```python
from build123d import *

# Parameters (mm, degrees)
BOSS_EXTRUDE4_DEPTH      = 3
SKETCH8_W                = 3
SKETCH8_H                = 8
SKETCH8_H_2              = 14.11
CUT_EXTRUDE5_DEPTH       = 3
SKETCH9_R                = 0.75
SKETCH9_W                = 12
SKETCH9_H                = 23.5
CUT_EXTRUDE6_DEPTH       = 3
FILLET2_R                = 5
SPLIT1_SURFACE_1_1_BACK  = 91.82
SPLIT1_SURFACE_1_1_DEPTH = 183.64
SPLIT1_SURFACE_1_2_BACK  = 91.82
SPLIT1_SURFACE_1_2_DEPTH = 183.64
SPLIT1_SURFACE_2_3_BACK  = 91.82
SPLIT1_SURFACE_2_3_DEPTH = 183.64
SPLIT1_SURFACE_2_4_BACK  = 91.82
SPLIT1_SURFACE_2_4_DEPTH = 183.64
SPLIT1_SURFACE_3_5_BACK  = 91.82
SPLIT1_SURFACE_3_5_DEPTH = 183.64
SPLIT1_SURFACE_3_6_BACK  = 91.82
SPLIT1_SURFACE_3_6_DEPTH = 183.64
SPLIT1_SURFACE_4_7_BACK  = 91.82
SPLIT1_SURFACE_4_7_DEPTH = 183.64
SPLIT1_SURFACE_4_8_BACK  = 91.82
SPLIT1_SURFACE_4_8_DEPTH = 183.64
SKETCH11_R               = 3
CUT_EXTRUDE7_DEPTH       = 10


with BuildPart() as part:
    # Sketch6 → Boss-Extrude4 (new body)
    with BuildSketch(Plane(origin=(0, 0, 0), x_dir=(1, 0, 0), z_dir=(0, 1, 0))):
        Polygon((-34.4, 16.055), (0, 30), (34.4, 16.055), (34.4, -16.055), (0, -30), (-34.4, -16.055), align=None)
    extrude(amount=BOSS_EXTRUDE4_DEPTH)

    # Sketch8 → Cut-Extrude5 (cut)
    with BuildSketch(Plane(origin=(0, 3, 0), x_dir=(1, 0, 0), z_dir=(0, 1, 0))):
        with Locations((32.9, 12.055)):
            Rectangle(SKETCH8_W, SKETCH8_H)
        with Locations((32.9, -9)):
            Rectangle(SKETCH8_W, SKETCH8_H_2)
        with Locations((-32.9, -9)):
            Rectangle(SKETCH8_W, SKETCH8_H_2)
        with Locations((-32.9, 12.055)):
            Rectangle(SKETCH8_W, SKETCH8_H)
    extrude(amount=-CUT_EXTRUDE5_DEPTH, mode=Mode.SUBTRACT)

    # Sketch9 → Cut-Extrude6 (cut)
    with BuildSketch(Plane(origin=(0, 3, 0), x_dir=(1, 0, 0), z_dir=(0, 1, 0))):
        with Locations(Location((-16.7, 16.555, 0), (0, 0, 270))):
            Circle(SKETCH9_R)
        with Locations(Location((-16.7, -10.445, 0), (0, 0, 90))):
            Circle(SKETCH9_R)
        with Locations((-16.7, 3.055)):
            Rectangle(SKETCH9_W, SKETCH9_H)
    extrude(amount=-CUT_EXTRUDE6_DEPTH, mode=Mode.SUBTRACT)

    # Fillet2
    fillet2_edges = [part.edges().sort_by_distance(p)[0] for p in [
        (0, 1.5, -30),
        (0, 1.5, 30),
    ]]
    fillet(fillet2_edges, radius=FILLET2_R)


with BuildPart() as body_2:
    # Split1: the piece behind the surface
    add(part.part)
    # Split1 surface 1: a surface, the sketch's curves swept straight by 183.64 mm
    with BuildLine(Plane(origin=(0, 3, 0), x_dir=(1, 0, 0), z_dir=(0, 1, 0)).offset(-SPLIT1_SURFACE_1_1_BACK), mode=Mode.PRIVATE) as split1_surface_1_1_path:
        Line((34.4, 16.055), (31.4, 16.055))
        Line((31.4, 16.055), (31.4, 17.271133721))
        Line((31.4, 17.271133721), (34.4, 16.055))
    split1_surface_1_1 = Shell.extrude(split1_surface_1_1_path.wire(), (0 * SPLIT1_SURFACE_1_1_DEPTH, 1 * SPLIT1_SURFACE_1_1_DEPTH, 0 * SPLIT1_SURFACE_1_1_DEPTH))
    split(bisect_by=split1_surface_1_1, keep=Keep.BOTTOM)


with BuildPart() as part_1:
    add(part.part)

    # Split1: split by a surface, the side it looks to stays
    # Split1 surface 1: a surface, the sketch's curves swept straight by 183.64 mm
    with BuildLine(Plane(origin=(0, 3, 0), x_dir=(1, 0, 0), z_dir=(0, 1, 0)).offset(-SPLIT1_SURFACE_1_2_BACK), mode=Mode.PRIVATE) as split1_surface_1_2_path:
        Line((34.4, 16.055), (31.4, 16.055))
        Line((31.4, 16.055), (31.4, 17.271133721))
        Line((31.4, 17.271133721), (34.4, 16.055))
    split1_surface_1_2 = Shell.extrude(split1_surface_1_2_path.wire(), (0 * SPLIT1_SURFACE_1_2_DEPTH, 1 * SPLIT1_SURFACE_1_2_DEPTH, 0 * SPLIT1_SURFACE_1_2_DEPTH))
    split(bisect_by=split1_surface_1_2, keep=Keep.TOP)


with BuildPart() as body_3:
    # Split1 2: the piece behind the surface
    add(part_1.part)
    # Split1 surface 2: a surface, the sketch's curves swept straight by 183.64 mm
    with BuildLine(Plane(origin=(0, 3, 0), x_dir=(1, 0, 0), z_dir=(0, 1, 0)).offset(-SPLIT1_SURFACE_2_3_BACK), mode=Mode.PRIVATE) as split1_surface_2_3_path:
        Line((31.4, -17.271133721), (31.4, -16.055))
        Line((31.4, -16.055), (34.4, -16.055))
        Line((34.4, -16.055), (31.4, -17.271133721))
    split1_surface_2_3 = Shell.extrude(split1_surface_2_3_path.wire(), (0 * SPLIT1_SURFACE_2_3_DEPTH, 1 * SPLIT1_SURFACE_2_3_DEPTH, 0 * SPLIT1_SURFACE_2_3_DEPTH))
    split(bisect_by=split1_surface_2_3, keep=Keep.BOTTOM)


with BuildPart() as part_2:
    add(part_1.part)

    # Split1 2: split by a surface, the side it looks to stays
    # Split1 surface 2: a surface, the sketch's curves swept straight by 183.64 mm
    with BuildLine(Plane(origin=(0, 3, 0), x_dir=(1, 0, 0), z_dir=(0, 1, 0)).offset(-SPLIT1_SURFACE_2_4_BACK), mode=Mode.PRIVATE) as split1_surface_2_4_path:
        Line((31.4, -17.271133721), (31.4, -16.055))
        Line((31.4, -16.055), (34.4, -16.055))
        Line((34.4, -16.055), (31.4, -17.271133721))
    split1_surface_2_4 = Shell.extrude(split1_surface_2_4_path.wire(), (0 * SPLIT1_SURFACE_2_4_DEPTH, 1 * SPLIT1_SURFACE_2_4_DEPTH, 0 * SPLIT1_SURFACE_2_4_DEPTH))
    split(bisect_by=split1_surface_2_4, keep=Keep.TOP)


with BuildPart() as body_4_2:
    # Split1 3: the piece behind the surface
    add(part_2.part)
    # Split1 surface 3: a surface, the sketch's curves swept straight by 183.64 mm
    with BuildLine(Plane(origin=(0, 3, 0), x_dir=(1, 0, 0), z_dir=(0, 1, 0)).offset(-SPLIT1_SURFACE_3_5_BACK), mode=Mode.PRIVATE) as split1_surface_3_5_path:
        Line((-31.4, -17.271133721), (-31.4, -16.055))
        Line((-31.4, -16.055), (-34.4, -16.055))
        Line((-34.4, -16.055), (-31.4, -17.271133721))
    split1_surface_3_5 = Shell.extrude(split1_surface_3_5_path.wire(), (0 * SPLIT1_SURFACE_3_5_DEPTH, 1 * SPLIT1_SURFACE_3_5_DEPTH, 0 * SPLIT1_SURFACE_3_5_DEPTH))
    split(bisect_by=split1_surface_3_5, keep=Keep.BOTTOM)


with BuildPart() as part_3:
    add(part_2.part)

    # Split1 3: split by a surface, the side it looks to stays
    # Split1 surface 3: a surface, the sketch's curves swept straight by 183.64 mm
    with BuildLine(Plane(origin=(0, 3, 0), x_dir=(1, 0, 0), z_dir=(0, 1, 0)).offset(-SPLIT1_SURFACE_3_6_BACK), mode=Mode.PRIVATE) as split1_surface_3_6_path:
        Line((-31.4, -17.271133721), (-31.4, -16.055))
        Line((-31.4, -16.055), (-34.4, -16.055))
        Line((-34.4, -16.055), (-31.4, -17.271133721))
    split1_surface_3_6 = Shell.extrude(split1_surface_3_6_path.wire(), (0 * SPLIT1_SURFACE_3_6_DEPTH, 1 * SPLIT1_SURFACE_3_6_DEPTH, 0 * SPLIT1_SURFACE_3_6_DEPTH))
    split(bisect_by=split1_surface_3_6, keep=Keep.TOP)


with BuildPart() as body_5_2:
    # Split1 4 body 4 2: the piece behind the surface
    add(body_4_2.part)
    # Split1 surface 4: a surface, the sketch's curves swept straight by 183.64 mm
    with BuildLine(Plane(origin=(0, 3, 0), x_dir=(1, 0, 0), z_dir=(0, 1, 0)).offset(-SPLIT1_SURFACE_4_7_BACK), mode=Mode.PRIVATE) as split1_surface_4_7_path:
        Line((-34.4, 16.055), (-31.4, 16.055))
        Line((-31.4, 16.055), (-31.4, 17.271133721))
        Line((-31.4, 17.271133721), (-34.4, 16.055))
    split1_surface_4_7 = Shell.extrude(split1_surface_4_7_path.wire(), (0 * SPLIT1_SURFACE_4_7_DEPTH, 1 * SPLIT1_SURFACE_4_7_DEPTH, 0 * SPLIT1_SURFACE_4_7_DEPTH))
    split(bisect_by=split1_surface_4_7, keep=Keep.BOTTOM)


with BuildPart() as body_4_2_1:
    add(body_4_2.part)

    # Split1 4 body 4 2: split by a surface, the side it looks to stays
    # Split1 surface 4: a surface, the sketch's curves swept straight by 183.64 mm
    with BuildLine(Plane(origin=(0, 3, 0), x_dir=(1, 0, 0), z_dir=(0, 1, 0)).offset(-SPLIT1_SURFACE_4_8_BACK), mode=Mode.PRIVATE) as split1_surface_4_8_path:
        Line((-34.4, 16.055), (-31.4, 16.055))
        Line((-31.4, 16.055), (-31.4, 17.271133721))
        Line((-31.4, 17.271133721), (-34.4, 16.055))
    split1_surface_4_8 = Shell.extrude(split1_surface_4_8_path.wire(), (0 * SPLIT1_SURFACE_4_8_DEPTH, 1 * SPLIT1_SURFACE_4_8_DEPTH, 0 * SPLIT1_SURFACE_4_8_DEPTH))
    split(bisect_by=split1_surface_4_8, keep=Keep.TOP)

    # Sketch11 → Cut-Extrude7 (cut)
    with BuildSketch(Plane(origin=(0, 3, 0), x_dir=(1, 0, 0), z_dir=(0, 1, 0))):
        with Locations(Location((16.7, -2.571133721, 0), (0, 0, 270))):
            Circle(SKETCH11_R)
    extrude(amount=-CUT_EXTRUDE7_DEPTH, mode=Mode.SUBTRACT)


solid = body_4_2_1.part
```
Build history of the part. All positions in model axes, mm. A direction names the side the tool comes from. Round coordinates to 2 decimals unless told otherwise and drop trailing zeros. Loops run counter-clockwise (first coordinate to the right, second up) from the corner with the lowest first, then second, coordinate; pieces in that order, holes last.
Item 1: Drill centre lines: line 1 along X through (y, z) = (0.35, -11); line 2 along X through (y, z) = (0.5, -1.5); line 3 along X through (y, z) = (0.75, 1). Where is each one in solid material? Low to high.
Item 2: Which spindle directions (+Z, -Z, +X, -X, +Y, -Y) get a long thin tool onto all of the face, cutting with end or side? Do faces 5 (the face through (-31.4, 2, 10)), 6 (the face through (33, 2, -8.055)), 7 (the face through (-33, 2, -8.055)), 8 (the face through (33, 2, 1.945)). Say none if no direction does.
Item 3: Saw through at B-B (z = 3.5). List the corners of the cut face in (x, y), then the cut area to 3 significant figures.
Item 4: Saw through at D-D (x = 16.7). List the corners of the cut face in (y, z).
Item 5: Saw through at C-C (x = -16.7). List the corners of the cut face in (y, z) (3 decimals).
Item 6: Two-plate mould, pull along X, no slides. Class faces 1 (the face through (-16.85, 1.48, -23.17)), 2 (the face through (31.4, 1, 10)), 3 (the face through (-16.667, 1.521, -17.304)), 4 (the face through (-17, 2, 8.695)): released by +X, released by -X, zero draft, split by the parting line, or undercut.
Item 7: Saw through at A-A (y = 2.2). List the corners of the cut face in (x, z) (3 decimals).
Item 8: Pin check, flat tips, straight feed: P1, Ø0.9, axis at y = 1.5, z = -14.5, coming from the -X side; P2, Ø5, axis at x = 16.7, z = 2.57, coming from the +Y side; P3, Ø1.5, axis at x = -15.5, y = 2, coming from the -Z side; P4, Ø0.9, axis at x = -33, y = 1.5, coming from the -Z side (3 decimals). Stop position of each tip, or through.
Worked answers:
1. line 1: x = -31.4 to -22.7, -10.7 to 31.4
1. line 2: x = -34.4 to -22.7, -10.7 to 34.4
1. line 3: x = -34.4 to -22.7, -10.7 to 14.14, 19.26 to 34.4
2. face 5: +Z, -X, +Y, -Y
2. face 6: -Z, +X, +Y, -Y
2. face 7: -Z, -X, +Y, -Y
2. face 8: +Z, +X, +Y, -Y
3. outline: (-31.4, 0) - (-22.7, 0) - (-22.7, 3) - (-31.4, 3) - close; (-10.7, 0) - (13.85, 0) - (13.85, 3) - (-10.7, 3) - close; (19.55, 0) - (31.4, 0) - (31.4, 3) - (19.55, 3) - close
3. area: 135 mm2
4. outline: (0, -23.23) - (3, -23.23) - (3, -0.43) - (0, -0.43) - close; (0, 5.57) - (3, 5.57) - (3, 23.23) - (0, 23.23) - close
5. outline: (0, -23.23) - (3, -23.23) - (3, -17.305) - (0, -17.305) - close; (0, -15.805) - (3, -15.805) - (3, -14.805) - (0, -14.805) - close; (0, 8.695) - (3, 8.695) - (3, 9.695) - (0, 9.695) - close; (0, 11.195) - (3, 11.195) - (3, 23.23) - (0, 23.23) - close
6. face 1: released by -X
6. face 2: released by +X
6. face 3: undercut
6. face 4: undercut
7. outline: (-34.4, -8.055) - (-31.4, -8.055) - (-31.4, -17.271) - (-1.878, -29.239) arc R5 ccw to (1.878, -29.239) - (31.4, -17.271) - (31.4, -8.055) - (34.4, -8.055) - (34.4, 1.945) - (31.4, 1.945) - (31.4, 17.271) - (1.878, 29.239) arc R5 ccw to (-1.878, 29.239) - (-31.4, 17.271) - (-31.4, 1.945) - (-34.4, 1.945) - close; hole (-22.7, -14.805) - (-10.7, -14.805) - (-10.7, 8.695) - (-22.7, 8.695) - close; hole circle Ø1.5 at (-16.7, -16.555); hole circle Ø1.5 at (-16.7, 10.445); hole circle Ø6 at (16.7, 2.571)
8. P1: stops at x = -31.4
8. P2: passes through
8. P3: stops at z = -24.02
8. P4: stops at z = -8.055
